```python
from build123d import *

# Parameters (mm, degrees)
F0_R      = 76.2
F1_DEPTH  = 25.4
F2_R      = 76.2
F2_R_2    = 50.8
F3_DEPTH  = 25.4
F4_R      = 6.35
F5_DEPTH  = 162.814
F6_W      = 177.8
F6_H      = 177.8
F7_DEPTH  = 25.4
F8_R      = 6.35
F9_DEPTH  = 67.818
F10_W     = 38.1
F10_H     = 38.1
F11_DEPTH = 38.1
F12_SIZE  = 5.08
F13_SIZE  = 5.08


with BuildPart() as f1:
    # F0 (on Top) → F1 (new body)
    with BuildSketch(Plane.XY):
        Circle(F0_R)
    extrude(amount=F1_DEPTH)

    # F2 (on face) → F3 (join)
    with BuildSketch(Plane.XY.offset(25.4)):
        Circle(F2_R)
        Circle(F2_R_2, mode=Mode.SUBTRACT)
    extrude(amount=F3_DEPTH)

    # F4 (on face) → F5 (cut)
    with BuildSketch(Plane.XY.offset(25.4)):
        Circle(F4_R)
    extrude(amount=-F5_DEPTH, mode=Mode.SUBTRACT)

    # F6 (on face) → F7 (join)
    with BuildSketch(Plane(origin=(0, 0, 0), x_dir=(1, 0, 0), z_dir=(0, 0, -1))):
        Rectangle(F6_W, F6_H)
    extrude(amount=F7_DEPTH)

    # F8 (on face) → F9 (cut)
    with BuildSketch(Plane(origin=(0, 0, -25.4), x_dir=(1, 0, 0), z_dir=(0, 0, -1))):
        Circle(F8_R)
    extrude(amount=-F9_DEPTH, mode=Mode.SUBTRACT)

    # F10 (on face) → F11 (join)
    with BuildSketch(Plane(origin=(0, 0, -25.4), x_dir=(1, 0, 0), z_dir=(0, 0, -1))):
        with Locations((-69.85, 69.85)):
            Rectangle(F10_W, F10_H)
        with Locations((-69.85, -69.85)):
            Rectangle(F10_W, F10_H)
        with Locations((69.85, 69.85)):
            Rectangle(F10_W, F10_H)
        with Locations((69.85, -69.85)):
            Rectangle(F10_W, F10_H)
    extrude(amount=F11_DEPTH)

    # F12
    f12_edges = [f1.edges().sort_by_distance(p)[0] for p in [
        (0, -88.9, 0),
        (-88.9, 0, 0),
        (88.9, 0, 0),
        (0, 88.9, 0),
        (88.9, -88.9, -31.75),
        (69.85, -88.9, -63.5),
        (50.8, -88.9, -44.45),
        (0, -88.9, -25.4),
        (-50.8, -88.9, -44.45),
        (-69.85, -88.9, -63.5),
        (-88.9, -88.9, -31.75),
        (-88.9, -69.85, -63.5),
        (-88.9, -50.8, -44.45),
        (-88.9, 0, -25.4),
        (-88.9, 50.8, -44.45),
        (-88.9, 69.85, -63.5),
        (-88.9, 88.9, -31.75),
        (-69.85, 88.9, -63.5),
        (-50.8, 88.9, -44.45),
        (0, 88.9, -25.4),
        (50.8, 88.9, -44.45),
        (69.85, 88.9, -63.5),
        (88.9, 88.9, -31.75),
        (88.9, 69.85, -63.5),
        (88.9, 50.8, -44.45),
        (88.9, 0, -25.4),
        (88.9, -50.8, -44.45),
        (88.9, -69.85, -63.5),
    ]]
    chamfer(f12_edges, length=F12_SIZE)

    # F13
    f13_edges = [f1.edges().sort_by_distance(p)[0] for p in [
        (-50.8, -67.31, -63.5),
        (-67.31, -50.8, -63.5),
        (50.8, -67.31, -63.5),
        (67.31, -50.8, -63.5),
        (-67.31, 50.8, -63.5),
        (-50.8, 67.31, -63.5),
        (67.31, 50.8, -63.5),
        (50.8, 67.31, -63.5),
    ]]
    chamfer(f13_edges, length=F13_SIZE)


solid = f1.part
```
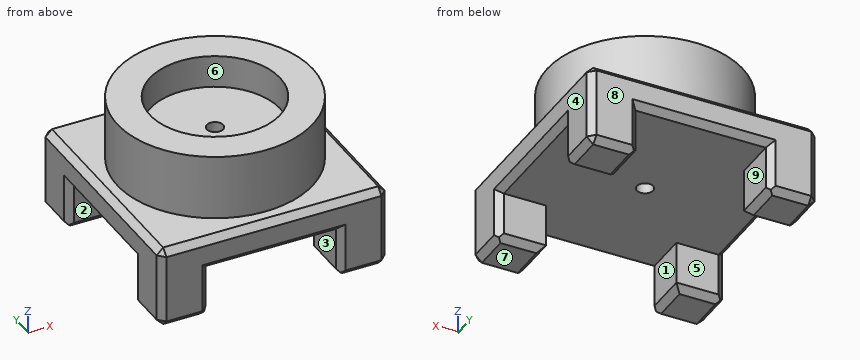
Input: part model. Units: mm. Frame: model coordinates. Face numbers are marked on the shaded views. A direction names the side the tool comes from. Coordinates: 2 decimals unless noted, no trailing zeros. Write each loop counter-clockwise with the first axis right and the second up, starting at its lowest first coordinate (ties: lowest second). Pieces come first, ordered by that corner, then holes. Notation, with made-up numbers: (33, -19.75) -> (86, -19.75) arc R22 ccw to (86, 7.25) -> close; hole circle Ø1 at (72, -30). An arc over 180 degrees is marked (long way). Answer as a JSON object with one key per item and string values.
1. Access query for the marked faces 5, 6, 7, 8 and 9. Directions: +Z, -Z, +X, -X, +Y, -Y. A direction counts if a zero-diameter tool reaches every point of the face in a straight line with its end or side. Return the directions, or none.
Result set:
{"face 5": "-Z, +X, -X", "face 6": "+Z", "face 7": "-Z, +X, -X, +Y, -Y", "face 8": "+Z, -Z, +X, -X, +Y", "face 9": "-Z, +Y, -Y"}
2. Section B-B on y = 0. Return the cut outline in (x, z).
Result set:
{"outline": "(-88.9, -20.32) -> (-83.82, -25.4) -> (-6.35, -25.4) -> (-6.35, 25.4) -> (-50.8, 25.4) -> (-50.8, 50.8) -> (-76.2, 50.8) -> (-76.2, 0) -> (-83.82, 0) -> (-88.9, -5.08) -> close; (6.35, -25.4) -> (83.82, -25.4) -> (88.9, -20.32) -> (88.9, -5.08) -> (83.82, 0) -> (76.2, 0) -> (76.2, 50.8) -> (50.8, 50.8) -> (50.8, 25.4) -> (6.35, 25.4) -> close"}
3. Section A-A on z = -54. Return the cut outline in (x, y), then the cut area to 3 significant figures.
Result set:
{"outline": "(-88.9, -83.82) -> (-83.82, -88.9) -> (-55.88, -88.9) -> (-50.8, -83.82) -> (-50.8, -50.8) -> (-83.82, -50.8) -> (-88.9, -55.88) -> close; (-88.9, 55.88) -> (-83.82, 50.8) -> (-50.8, 50.8) -> (-50.8, 83.82) -> (-55.88, 88.9) -> (-83.82, 88.9) -> (-88.9, 83.82) -> close; (50.8, -83.82) -> (55.88, -88.9) -> (83.82, -88.9) -> (88.9, -83.82) -> (88.9, -55.88) -> (83.82, -50.8) -> (50.8, -50.8) -> close; (50.8, 50.8) -> (83.82, 50.8) -> (88.9, 55.88) -> (88.9, 83.82) -> (83.82, 88.9) -> (55.88, 88.9) -> (50.8, 83.82) -> close", "area": "5,650 mm2"}
4. First-contact query: P1, Ø3, axis at x = 68, y = 5, coming from the -Z side; P2, Ø1, axis at x = 4.5, y = 43, coming from the +Z side; P3, Ø6, axis at y = -66, z = 31.5, coming from the -X side. Flat tips, straight axial feed; report the tip coordinate or a pass-through.
Result set:
{"P1": "stops at z = -25.4", "P2": "stops at z = 25.4", "P3": "stops at x = -42.87"}
5. Section D-D on x = 36.5. Return the cut outline in (y, z).
Result set:
{"outline": "(-88.9, -20.32) -> (-83.82, -25.4) -> (83.82, -25.4) -> (88.9, -20.32) -> (88.9, -5.08) -> (83.82, 0) -> (66.89, 0) -> (66.89, 50.8) -> (35.33, 50.8) -> (35.33, 25.4) -> (-35.33, 25.4) -> (-35.33, 50.8) -> (-66.89, 50.8) -> (-66.89, 0) -> (-83.82, 0) -> (-88.9, -5.08) -> close"}
6. Mould query, pull axis X, two halves, no side actions, for the marked faces 1, 2, 3 and 4. Classes: released by +X, released by -X, zero draft, split by the parting line, or undercut.
Result set:
{"face 1": "undercut", "face 2": "zero draft", "face 3": "undercut", "face 4": "released by +X"}
7. Material intervals for line 1 (X direction, y = 0, z = -2.5); line 2 (X direction, y = -79.5, z = -31); line 3 (Y direction, x = 0, z = 43), sorted ascending. Write a range as from..to.
Result set:
{"line 1": "x = -86.32..-6.35, 6.35..86.32", "line 2": "x = -88.9..-50.8, 50.8..88.9", "line 3": "y = -76.2..-50.8, 50.8..76.2"}
